Autodesk Inventor part; units mm, degrees
ref_plane "YZ Plane" through (0, 0, 0) normal (1, 0, 0) x (0, 1, 0)
ref_plane "XZ Plane" through (0, 0, 0) normal (0, 1, 0) x (-1, 0, 0)
ref_plane "XY Plane" through (0, 0, 0) normal (0, 0, 1) x (1, 0, 0)
sketch "Sketch1" plane through (0, 0, 0) normal (0, 0, 1) x (1, 0, 0)
  line L0 (0, 0) -> (0, -76.2)
  line L1 (0, -76.2) -> (25.4, -76.2)
  line L2 (25.4, -76.2) -> (76.2, -25.4)
  line L3 (76.2, -25.4) -> (76.2, 0)
  line L4 (76.2, 0) -> (0, 0)
  line L5 (12.7, -76.2) -> (12.7, 0) construction
  line L6 (0, -12.7) -> (76.2, -12.7) construction
  circle A0 centre (12.7, -12.7) radius 3.3734
  circle A1 centre (12.7, -38.1) radius 3.3734
  circle A2 centre (12.7, -63.5) radius 3.3734
  circle A3 centre (38.1, -12.7) radius 3.3734
  circle A4 centre (63.5, -12.7) radius 3.3734
  dimension "d0" = 76.2
  dimension "d1" = 25.4
  dimension "d2" = 12.7
  dimension "d3" = 6.7469
  dimension "d4" = 6.7469
  dimension "d5" = 6.7469
  dimension "d6" = 6.7469
  dimension "d7" = 6.7469
  dimension "d8" = 63.5
  dimension "d9" = 25.4
  dimension "d10" = 25.4
  dimension "d11" = 25.4
extrude "Extrusion1" add sketch "Sketch1" along normal blind 3.175
properties part number "gusset"
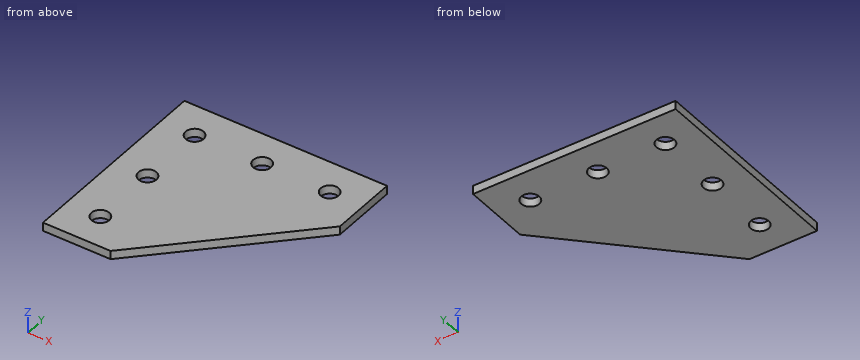
Part model, mm, in its own coordinate system. Round coordinates to 2 decimals unless told otherwise and drop trailing zeros. Order: outer loops, then holes, each group sorted by start corner. A loop starts at its lowest first (then second) coordinate and runs counter-clockwise, first axis right, second up. Notation, with made-up numbers: M 6,39.25 L 62,39.25 A10 cw 62,54.25 Z; hole C 8,69.25 d3. An arc over 180 degrees is marked long. Put each result on its own line as item: value. Start each with the question number.
1. Slice it at D-D on x = 63.5. List the corners of the cut face in (y, z) (3 decimals).
2. Slice it at B-B on x = 12.7. List the corners of the cut face in (y, z) (3 decimals).
3. Slice it at C-C on z = 1.3. List the corners of the cut face in (x, y).
4. Slice it at A-A on y = -12.7. List the corners of the cut face in (x, z) (3 decimals), then the cut area to 3 significant figures.
5. Drill centre lines: probe 1 along Y at (x, z) = (12.7, 2); probe 2 along Y at (x, z) = (63.5, 2.1); probe 3 along Y at (x, z) = (60.5, 1.2). Where is each one in solid material? Low to high. Write a range as [from, to].
Findings:
1. outline: M -38.1,0 L -16.073,0 L -16.073,3.175 L -38.1,3.175 Z; M -9.327,0 L 0,0 L 0,3.175 L -9.327,3.175 Z
2. outline: M -76.2,0 L -66.873,0 L -66.873,3.175 L -76.2,3.175 Z; M -60.127,0 L -41.473,0 L -41.473,3.175 L -60.127,3.175 Z; M -34.727,0 L -16.073,0 L -16.073,3.175 L -34.727,3.175 Z; M -9.327,0 L 0,0 L 0,3.175 L -9.327,3.175 Z
3. outline: M 0,-76.2 L 25.4,-76.2 L 76.2,-25.4 L 76.2,0 L 0,0 Z; hole C 12.7,-63.5 d6.75; hole C 12.7,-38.1 d6.75; hole C 12.7,-12.7 d6.75; hole C 38.1,-12.7 d6.75; hole C 63.5,-12.7 d6.75
4. outline: M 0,0 L 9.327,0 L 9.327,3.175 L 0,3.175 Z; M 16.073,0 L 34.727,0 L 34.727,3.175 L 16.073,3.175 Z; M 41.473,0 L 60.127,0 L 60.127,3.175 L 41.473,3.175 Z; M 66.873,0 L 76.2,0 L 76.2,3.175 L 66.873,3.175 Z
4. area: 178 mm2
5. probe 1: [-76.2, -66.87], [-60.13, -41.47], [-34.73, -16.07], [-9.33, 0]
5. probe 2: [-38.1, -16.07], [-9.33, 0]
5. probe 3: [-41.1, -14.24], [-11.16, 0]
